Part model, mm, in its own coordinate system. A direction names the side the tool comes from. Round coordinates to 2 decimals unless told otherwise and drop trailing zeros. Loops run counter-clockwise (first coordinate to the right, second up) from the corner with the lowest first, then second, coordinate; pieces in that order, holes last. Notation, with made-up numbers: (-7.75, 12.5) -> (8.25, 12.5) arc R23 ccw to (8.25, 28.5) -> close; hole circle Ø11 at (-8, 82.5). An arc over 180 degrees is marked (long way). Use a Markdown table: item, result. Add a question column.
Item 1: Cut at C-C, the plane y = -2.5. List the corners of the cut face in (x, z), plus the area to 3 significant figures.
Item 2: Cut at A-A, the plane x = 0. List the corners of the cut face in (y, z), plus the area to 3 significant figures.
Item 3: Probe line 1 (X direction, y = 6, z = 6); line 2 (Y direction, x = -1.75, z = 8); line 3 (Z direction, x = -1, y = 1.5). List the from-to ranges inside material, lowest first. Write a range as [from, to].
Item 4: Two-plate mould, pull along Z, no slides. Class faces 1 (the face through (-12, -5, 15)), 2 (the face through (0, 0, -1.5)), 3 (the face through (0, 6.5, 7)), 4 (the face through (7.7, -7.507, 12.993)): pulls with the +Z half, pulls with the -Z half, needs draft (parallel to the pull), parting line crosses it, or undercut.
Item 5: Cut at D-D, the plane x = -5.75. List the corners of the cut face in (y, z), plus the area to 3 significant figures.
Item 6: Flat gauge pins, fed straight in: pin 1 (4 mm diameter, centred on x = 3.5, y = 3, fed in from +Z); pin 2 (1.1 mm diameter, centred on x = -12, y = -4.5, fed in from +Z); pin 3 (1.2 mm diameter, centred on x = -12.5, y = -1, fed in from +Z). Where does each tip first touch, or does it go through?
Item 7: Which spindle directions (+Z, -Z, +X, -X, +Y, -Y) get a long thin tool onto all of the face, cutting with end or side? Do faces 5 (the face through (-12, -3.5, 9)), 6 (the face through (-7.7, -7.507, 7.007)), 7 (the face through (11.5, 0, 7)), 8 (the face through (3, 7, 15)). Say none if no direction does.
Item 8: Cut at B-B, the plane z = 4.25. List the corners of the cut face in (x, y), plus the area to 3 significant figures.
```python
from build123d import *

# Parameters (mm, degrees)
F1_DEPTH = 15
F0_W     = 1.5
F0_H     = 7
F2_DEPTH = 1.5
F4_DEPTH = 6
F5_DEPTH = 3
F7_DEPTH = 1
F8_R     = 0.5


with BuildPart() as f1:
    # F0 (on Top) → F1 (new body)
    with BuildSketch(Plane.XY):
        Polygon((13, -8), (13, 8), (-13, 8), (-13, 3.5), (-11.5, 3.5), (-11.5, 6.5), (11.5, 6.5), (11.5, -6.5), (-11.5, -6.5), (-11.5, -3.5), (-13, -3.5), (-13, -8), align=None)
    extrude(amount=F1_DEPTH)

    # F0 (on Top) → F2 (join)
    with BuildSketch(Plane.XY):
        Polygon((-11.5, 6.5), (-11.5, 3.5), (-11.5, -3.5), (-11.5, -6.5), (11.5, -6.5), (11.5, 6.5), align=None)
        Polygon((13, -8), (13, 8), (-13, 8), (-13, 3.5), (-11.5, 3.5), (-11.5, 6.5), (11.5, 6.5), (11.5, -6.5), (-11.5, -6.5), (-11.5, -3.5), (-13, -3.5), (-13, -8), align=None)
        with Locations((-12.25, 0)):
            Rectangle(F0_W, F0_H)
    extrude(amount=-F2_DEPTH)

    # F3 (on face) → F4 (join)
    with BuildSketch(Plane.XY.offset(15)):
        Polygon((11.5, -6.5), (-11.5, -6.5), (-13, -6.5), (-13, -8), (13, -8), (13, -6.5), align=None)
    extrude(amount=F4_DEPTH)

    # F0 (on Top) → F5 (join)
    with BuildSketch(Plane.XY):
        with Locations((-12.25, 0)):
            Rectangle(F0_W, F0_H)
    extrude(amount=F5_DEPTH)

    # F6 (on face) → F7 (cut)
    with BuildSketch(Plane.XZ.offset(8)):
        with BuildLine():
            Line((-2.2407097466, 13.5), (2.25, 13.5))
            Line((2.25, 13.5), (2.25, 17))
            ThreePointArc((2.25, 17), (-0.0077226241, 19.2437825827), (-2.2515052067, 16.9860599586))
            Line((-2.2515052067, 16.9860599586), (-2.2407097466, 13.5))
        make_face()
        Polygon((13, 12.5), (2.25, 13.5), (-2.2407097466, 13.5), (-13, 12.5), (-13, 7.5), (-2.25, 6.5), (2.25, 6.5), (13, 7.5), align=None)
        with BuildLine():
            Line((2.25, 3), (2.25, 6.5))
            Line((2.25, 6.5), (-2.25, 6.5))
            Line((-2.25, 6.5), (-2.25, 3.5))
            ThreePointArc((-2.25, 3.5), (-0.25, 1), (2.25, 3))
        make_face()
    extrude(amount=-F7_DEPTH, mode=Mode.SUBTRACT)

    # F8
    f8_edges = [f1.edges().sort_by_distance(p)[0] for p in [
        (13, 0.75, 15),
        (0, 8, 15),
        (-13, 5.75, 15),
        (-13, -5, 15),
        (13, -6.5, 18),
        (0, -6.5, 21),
        (-13, -8, 3),
        (0, -8, -1.5),
        (-13, 0, -1.5),
        (13, 0, -1.5),
        (0, 8, -1.5),
        (13, 8, 6.75),
        (-13, 8, 6.75),
        (0, -8, 21),
        (-13, -8, 16.75),
        (-13, -6.5, 18),
        (13, -8, 16.75),
        (13, -8, 3),
    ]]
    fillet(f8_edges, radius=F8_R)


solid = f1.part
```
A:
| question | item | result |
|---|---|---|
| 1 | outline | (-13, -1) arc R0.5 ccw to (-12.5, -1.5) -> (12.5, -1.5) arc R0.5 ccw to (13, -1) -> (13, 14.5) arc R0.5 ccw to (12.5, 15) -> (11.5, 15) -> (11.5, 0) -> (-11.5, 0) -> (-11.5, 3) -> (-13, 3) -> close |
| 1 | area | 65.8 mm^2 |
| 2 | outline | (-8, -1) arc R0.5 ccw to (-7.5, -1.5) -> (7.5, -1.5) arc R0.5 ccw to (8, -1) -> (8, 14.5) arc R0.5 ccw to (7.5, 15) -> (6.5, 15) -> (6.5, 0) -> (-6.5, 0) -> (-6.5, 20.5) arc R0.5 ccw to (-7, 21) -> (-7.5, 21) arc R0.5 ccw to (-8, 20.5) -> (-8, 19.24) -> (-7, 19.24) -> (-7, 0.99) -> (-8, 0.99) -> close |
| 2 | area | 59.5 mm^2 |
| 3 | line 1 | x = [-13, -11.5], [11.5, 13] |
| 3 | line 2 | y = [-7, -6.5], [6.5, 8] |
| 3 | line 3 | z = [-1.5, 0] |
| 4 | face 1 | pulls with the +Z half |
| 4 | face 2 | pulls with the -Z half |
| 4 | face 3 | needs draft |
| 4 | face 4 | undercut |
| 5 | outline | (-8, -1) arc R0.5 ccw to (-7.5, -1.5) -> (7.5, -1.5) arc R0.5 ccw to (8, -1) -> (8, 14.5) arc R0.5 ccw to (7.5, 15) -> (6.5, 15) -> (6.5, 0) -> (-6.5, 0) -> (-6.5, 20.5) arc R0.5 ccw to (-7, 21) -> (-7.5, 21) arc R0.5 ccw to (-8, 20.5) -> (-8, 13.17) -> (-7, 13.17) -> (-7, 6.83) -> (-8, 6.83) -> close |
| 5 | area | 71.4 mm^2 |
| 6 | pin 1 | stops at z = 0 |
| 6 | pin 2 | stops at z = 15 |
| 6 | pin 3 | stops at z = 3 |
| 7 | face 5 | +Z, -X |
| 7 | face 6 | -Y |
| 7 | face 7 | +Z |
| 7 | face 8 | +Z, +X, -X, +Y |
| 8 | outline | (-13, -7.5) arc R0.5 ccw to (-12.5, -8) -> (-2.25, -8) -> (-2.25, -7) -> (2.25, -7) -> (2.25, -8) -> (12.5, -8) arc R0.5 ccw to (13, -7.5) -> (13, 7.5) arc R0.5 ccw to (12.5, 8) -> (-12.5, 8) arc R0.5 ccw to (-13, 7.5) -> (-13, 3.5) -> (-11.5, 3.5) -> (-11.5, 6.5) -> (11.5, 6.5) -> (11.5, -6.5) -> (-11.5, -6.5) -> (-11.5, -3.5) -> (-13, -3.5) -> close |
| 8 | area | 102 mm^2 |
